Geometry: final body of the model. Coordinates: model frame, mm. Face numbers are marked on the shaded views. A direction names the side the tool comes from. Coordinates: 2 decimals unless noted, no trailing zeros. Order: outer loops, then holes, each group sorted by start corner. A loop starts at its lowest first (then second) coordinate and runs counter-clockwise, first axis right, second up. Notation, with made-up numbers: (-14.5, 33) -> (0.5, 33) arc R11 ccw to (0.5, 39) -> close; hole circle Ø5 at (37.25, 47). An arc over 180 degrees is marked (long way). Answer in a Markdown table with one row per item. Add a question column.
1) Ray query, line 1 (Y direction, x = -4.5, z = 0.5); line 2 (X direction, y = -4, z = 0); line 3 (X direction, y = -8, z = -2). Return the intervals inside material, ascending. Write a range as from..to.
2) Section query C-C on y = -5.5. Return the cut outline in (x, z) (1 decimal), then the cut area to 3 significant figures.
3) Set-up query: the marked faces 4, 5 and 6. Return all of +Z, -Z, +X, -X, +Y, -Y with unobstructed straight access to the full face (end or side cutting, diameter ignored); none if empty.
4) Contact query for flat-ended pins moving along their axis: P1, Ø4, axis at x = -2, y = -1.5, coming from the -Z side; P2, Ø2, axis at x = -4.5, z = -1, coming from the +Y side; P3, Ø2, axis at x = -7.5, y = 0, coming from the -Z side. Output: stop coordinate, or through.
5) Section query B-B on z = 0. Return the cut outline in (x, y), then the cut area to 3 significant figures.
6) Section query D-D on y = 1. Return the cut outline in (x, z) (1 decimal).
7) Section query A-A on x = -3.75. Return the cut outline in (y, z), then the cut area to 3 significant figures.
8) Pull-direction query (Y, two-part tool) for the marked faces 1, 2 and 3; classes: +Y half, -Y half, draft (parallel to the pull), parting line (faces both ways), or undercut.
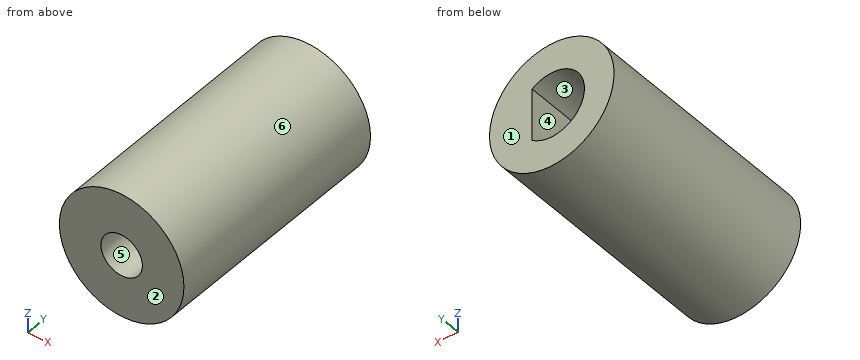
```python
from build123d import *

# Parameters (mm, degrees)
SKETCH1_R                = 4.7625
BOSS_EXTRUDE1_DEPTH      = 9
BOSS_EXTRUDE1_DEPTH_BACK = 9
CUT_EXTRUDE1_DEPTH       = 7
SKETCH7_R                = 1.5875
CUT_EXTRUDE2_DEPTH       = 7


with BuildPart() as part:
    # Sketch1 → Boss-Extrude1 (new body, two sides)
    with BuildSketch(Plane(origin=(0, 0, 0), x_dir=(1, 0, 0), z_dir=(0, 1, 0))) as boss_extrude1_sk:
        with Locations((-4.672198487, 0.923020882)):
            Circle(SKETCH1_R)
    extrude(amount=BOSS_EXTRUDE1_DEPTH)
    extrude(boss_extrude1_sk.sketch, amount=-BOSS_EXTRUDE1_DEPTH_BACK)

    # Sketch6 → Cut-Extrude1 (cut)
    with BuildSketch(Plane(origin=(0, 9, 0), x_dir=(1, 0, 0), z_dir=(0, 1, 0))):
        with BuildLine():
            Line((-3.172198487, -1.076979118), (-3.172198487, 2.923020882))
            ThreePointArc((-3.172198487, 2.923020882), (-7.172198487, 0.923020882), (-3.172198487, -1.076979118))
        make_face()
    extrude(amount=-CUT_EXTRUDE1_DEPTH, mode=Mode.SUBTRACT)

    # Sketch7 → Cut-Extrude2 (cut)
    with BuildSketch(Plane.XZ.offset(9)):
        with Locations((-4.672198487, -0.923020882)):
            Circle(SKETCH7_R)
    extrude(amount=-CUT_EXTRUDE2_DEPTH, mode=Mode.SUBTRACT)


solid = part.part
```
Result:
| question | item | result |
|---|---|---|
| 1 | line 1 | -2..2 |
| 1 | line 2 | -9.34..-5.96, -3.38..0 |
| 1 | line 3 | -9.31..-5.84, -3.51..-0.03 |
| 2 | outline | circle Ø9.5 at (-4.7, -0.9); hole circle Ø3.2 at (-4.7, -0.9) |
| 2 | area | 63.3 mm2 |
| 3 | face 4 | +Y |
| 3 | face 5 | -Y |
| 3 | face 6 | +Y, -Y |
| 4 | P1 | z = -5.64 |
| 4 | P2 | y = 2 |
| 4 | P3 | z = -5.32 |
| 5 | outline | (-9.34, -9) -> (-5.96, -9) -> (-5.96, -2) -> (-3.38, -2) -> (-3.38, -9) -> (0, -9) -> (0, 9) -> (-3.17, 9) -> (-3.17, 2) -> (-7, 2) -> (-7, 9) -> (-9.34, 9) -> close |
| 5 | area | 123 mm2 |
| 6 | outline | circle Ø9.5 at (-4.7, -0.9) |
| 7 | outline | (-9, -5.6) -> (9, -5.6) -> (9, -3.25) -> (2, -3.25) -> (2, 1.4) -> (9, 1.4) -> (9, 3.75) -> (-9, 3.75) -> (-9, 0.37) -> (-2, 0.37) -> (-2, -2.22) -> (-9, -2.22) -> close |
| 7 | area | 118 mm2 |
| 8 | face 1 | +Y half |
| 8 | face 2 | -Y half |
| 8 | face 3 | draft |
